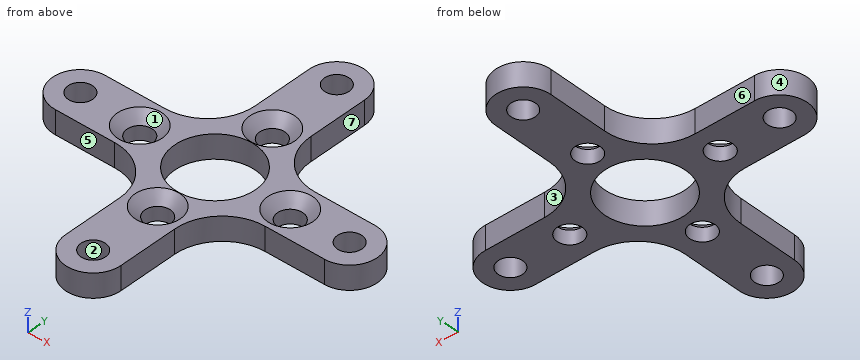
```python
from build123d import *

# Parameters (mm, degrees)
SKETCH1_R           = 5.1
SKETCH1_R_2         = 1.6
SKETCH1_R_3         = 1.55
BOSS_EXTRUDE1_DEPTH = 3
CHAMFER1_SIZE       = 1.25


with BuildPart() as part:
    # Sketch1 → Boss-Extrude1 (new body)
    with BuildSketch(Plane(origin=(0, 0, 0), x_dir=(0, 1, 0), z_dir=(0, 0, 1))):
        with BuildLine():
            Line((3.5, 17), (3.5, 9.5))
            ThreePointArc((3.5, 9.5), (5.257359313, 5.257359313), (9.5, 3.5))
            Line((9.5, 3.5), (17, 3.5))
            ThreePointArc((17, 3.5), (20.5, 0), (17, -3.5))
            Line((17, -3.5), (9.5, -3.5))
            ThreePointArc((9.5, -3.5), (5.257359313, -5.257359313), (3.5, -9.5))
            Line((3.5, -9.5), (3.5, -17))
            ThreePointArc((3.5, -17), (0, -20.5), (-3.5, -17))
            Line((-3.5, -17), (-3.5, -9.5))
            ThreePointArc((-3.5, -9.5), (-5.257359313, -5.257359313), (-9.5, -3.5))
            Line((-9.5, -3.5), (-17, -3.5))
            ThreePointArc((-17, -3.5), (-20.5, 0), (-17, 3.5))
            Line((-17, 3.5), (-9.5, 3.5))
            ThreePointArc((-9.5, 3.5), (-5.257359313, 5.257359313), (-3.5, 9.5))
            Line((-3.5, 9.5), (-3.5, 17))
            ThreePointArc((-3.5, 17), (0, 20.5), (3.5, 17))
        make_face()
        with Locations(Location((0, 0, 0), (0, 0, 270))):
            Circle(SKETCH1_R, mode=Mode.SUBTRACT)
        with Locations(Location((0, 9.5, 0), (0, 0, 270))):
            Circle(SKETCH1_R_2, mode=Mode.SUBTRACT)
        with Locations(Location((8, 0, 0), (0, 0, 270))):
            Circle(SKETCH1_R_2, mode=Mode.SUBTRACT)
        with Locations(Location((-8, 0, 0), (0, 0, 270))):
            Circle(SKETCH1_R_2, mode=Mode.SUBTRACT)
        with Locations(Location((0, -9.5, 0), (0, 0, 270))):
            Circle(SKETCH1_R_2, mode=Mode.SUBTRACT)
        with Locations(Location((0, 17, 0), (0, 0, 270))):
            Circle(SKETCH1_R_3, mode=Mode.SUBTRACT)
        with Locations(Location((17, 0, 0), (0, 0, 270))):
            Circle(SKETCH1_R_3, mode=Mode.SUBTRACT)
        with Locations(Location((-17, 0, 0), (0, 0, 270))):
            Circle(SKETCH1_R_3, mode=Mode.SUBTRACT)
        with Locations(Location((0, -17, 0), (0, 0, 270))):
            Circle(SKETCH1_R_3, mode=Mode.SUBTRACT)
    extrude(amount=BOSS_EXTRUDE1_DEPTH)

    # Chamfer1
    chamfer1_edges = [part.edges().sort_by_distance(p)[0] for p in [
        (-11.1, 0, 3),
        (-1.6, 8, 3),
        (-1.6, -8, 3),
        (7.9, 0, 3),
    ]]
    chamfer(chamfer1_edges, length=CHAMFER1_SIZE)


solid = part.part
```
Design review of the part built by this model. Coordinates are the model's own, in mm. Face numbers are marked on the shaded views. A direction names the side the tool comes from. Give positions to 0.01 mm unless a question says otherwise; leave off trailing zeros. Write each loop counter-clockwise with the first axis right and the second up, starting at its lowest first coordinate (ties: lowest second). Pieces come first, ordered by that corner, then holes. Notation, with made-up numbers: (65, 55) -> (113, 55) arc R17 cw to (113, 59) -> close; hole circle Ø6 at (43.5, -31.5). An arc over 180 degrees is marked (long way). Answer in a Markdown table with one row per item.
(1) Consider section B-B (z = 2.25). Count the separate pieces of the cut face and the enclosed holes in it, then the cut area to 3 significant figures.
Results:
| item | result |
|---|---|
| separate pieces | 1 |
| enclosed holes | 9 |
| area | 368 mm2 |
(2) To check wall thickness, follow probe 1 along Y at (x, z) = (0, 1.5); probe 2 along Y at (x, z) = (17, 1.05); probe 3 along Y at (x, z) = (-9.5, 1.35). State the ranges of each line that lie inside material, in increasing order.
Results:
| item | result |
|---|---|
| probe 1 | -20.5 to -18.55, -15.45 to -9.6, -6.4 to -5.1, 5.1 to 6.4, 9.6 to 15.45, 18.55 to 20.5 |
| probe 2 | -3.5 to -1.55, 1.55 to 3.5 |
| probe 3 | -3.5 to -1.6, 1.6 to 3.5 |
(3) Consider section A-A (y = 0). State the section outline as (x, z) points, then the cut area to 3 significant figures.
Results:
| item | result |
|---|---|
| outline | (-20.5, 0) -> (-18.55, 0) -> (-18.55, 3) -> (-20.5, 3) -> close; (-15.45, 0) -> (-11.1, 0) -> (-11.1, 1.75) -> (-12.35, 3) -> (-15.45, 3) -> close; (-7.9, 0) -> (-5.1, 0) -> (-5.1, 3) -> (-6.65, 3) -> (-7.9, 1.75) -> close; (5.1, 0) -> (7.9, 0) -> (7.9, 1.75) -> (6.65, 3) -> (5.1, 3) -> close; (11.1, 0) -> (15.45, 0) -> (15.45, 3) -> (12.35, 3) -> (11.1, 1.75) -> close; (18.55, 0) -> (20.5, 0) -> (20.5, 3) -> (18.55, 3) -> close |
| area | 51.5 mm2 |
(4) Mouldability with a two-part tool opening along X and no side actions: class the marked faces 1, 2, 3 and 4 as +X half, -X half, draft (parallel to the pull), parting line (faces both ways), or undercut.
Results:
| item | result |
|---|---|
| face 1 | undercut |
| face 2 | undercut |
| face 3 | +X half |
| face 4 | -X half |
(5) For the marked faces 5, 6 and 7, list the 3-axis set-ups (+Z, -Z, +X, -X, +Y, -Y) from which the entire face can be reached by the end or side of a thin tool; tool diameter is ignored.
Results:
| item | result |
|---|---|
| face 5 | +Z, -Z, -X, -Y |
| face 6 | +Z, -Z, -X, +Y |
| face 7 | +Z, -Z, +X, +Y |
(6) Consider section C-C (x = 0). State the section outline as (y, z) points.
Results:
| item | result |
|---|---|
| outline | (-20.5, 0) -> (-18.55, 0) -> (-18.55, 3) -> (-20.5, 3) -> close; (-15.45, 0) -> (-9.6, 0) -> (-9.6, 1.75) -> (-10.85, 3) -> (-15.45, 3) -> close; (-6.4, 0) -> (-5.1, 0) -> (-5.1, 3) -> (-5.15, 3) -> (-6.4, 1.75) -> close; (5.1, 0) -> (6.4, 0) -> (6.4, 1.75) -> (5.15, 3) -> (5.1, 3) -> close; (9.6, 0) -> (15.45, 0) -> (15.45, 3) -> (10.85, 3) -> (9.6, 1.75) -> close; (18.55, 0) -> (20.5, 0) -> (20.5, 3) -> (18.55, 3) -> close |
(7) Clearance check with flat-ended pins moving along their axes: pin 1 (12 mm diameter, centred on x = -10, y = -10.5, fed in from +Z); pin 2 (5 mm diameter, centred on x = 0, y = 8, fed in from +Z); pin 3 (1.5 mm diameter, centred on y = 11.5, z = 2, fed in from -X); pin 4 (4 mm diameter, centred on x = 9.5, y = 0, fed in from +Z). State where each tip first meets the part, or that it passes through.
Results:
| item | result |
|---|---|
| pin 1 | through |
| pin 2 | z = 2.65 |
| pin 3 | x = -3.5 |
| pin 4 | z = 2.15 |
(8) Consider section D-D (y = 8). State the section outline as (x, z) points, then the cut area to 3 significant figures.
Results:
| item | result |
|---|---|
| outline | (-3.69, 0) -> (-1.6, 0) -> (-1.6, 1.75) -> (-2.85, 3) -> (-3.69, 3) -> close; (1.6, 0) -> (3.69, 0) -> (3.69, 3) -> (2.85, 3) -> (1.6, 1.75) -> close |
| area | 11.0 mm2 |
